Answer from the drawing. Dimensions are ordinates in mm from the lowest x, y and z of the part. A direction names the side the tool comes from. Round coordinates to 2 decimals unless told otherwise and drop trailing zeros. Write each loop counter-clockwise with the first axis right and the second up, starting at its lowest first coordinate (ties: lowest second). Pieces come first, ordered by that corner, then holes.
1. Find section A-A (x = 45). Write down the section's boundary in (y, z), and give its area (3 significant figures).
2. Find section D-D (z = 16). Write down the section's boundary in (x, y), and give its area (3 significant figures).
3. Determine the mould class of the marked faces 6, 7 and 8 for opening direction Z: pulls with the +Z half, pulls with the -Z half, needs draft (parallel to the pull), parting line crosses it, or undercut.
4. Find section B-B (y = 10). Write down the section's boundary in (x, z), and give its area (3 significant figures).
5. Flat-ended cylindrical pins translate along their axes: pin 1 Ø11 at (x, z) = (48, 37) entering from +Y; pin 2 Ø1 at (x, z) = (13.5, 14.5) entering from -Y; pin 3 Ø8 at (x, z) = (45.5, 33) entering from -Y; pin 4 Ø12 at (x, z) = (56.5, 17.5) entering from -Y. Find the tip coordinate at first contact, or state that the pin passes through.
6. Find section C-C (z = 34). Write down the section's boundary in (x, y).
7. Straight lines are drawn through the part: probe 1 along Z at (x, y) = (36, 8); probe 2 along X at (y, z) = (7.75, 8.5); probe 3 along X at (y, z) = (16.75, 16). For each, find the intervals that lie inside material, in ascending order.
8. A tool of negligible diameter and unlimited length cuts with its end or side. For the marked faces 1, 2, 3, 4 and 5, from which of +Z, -Z, +X, -X, +Y, -Y can it reach the whole face along a straight path? Write none if from no direction.
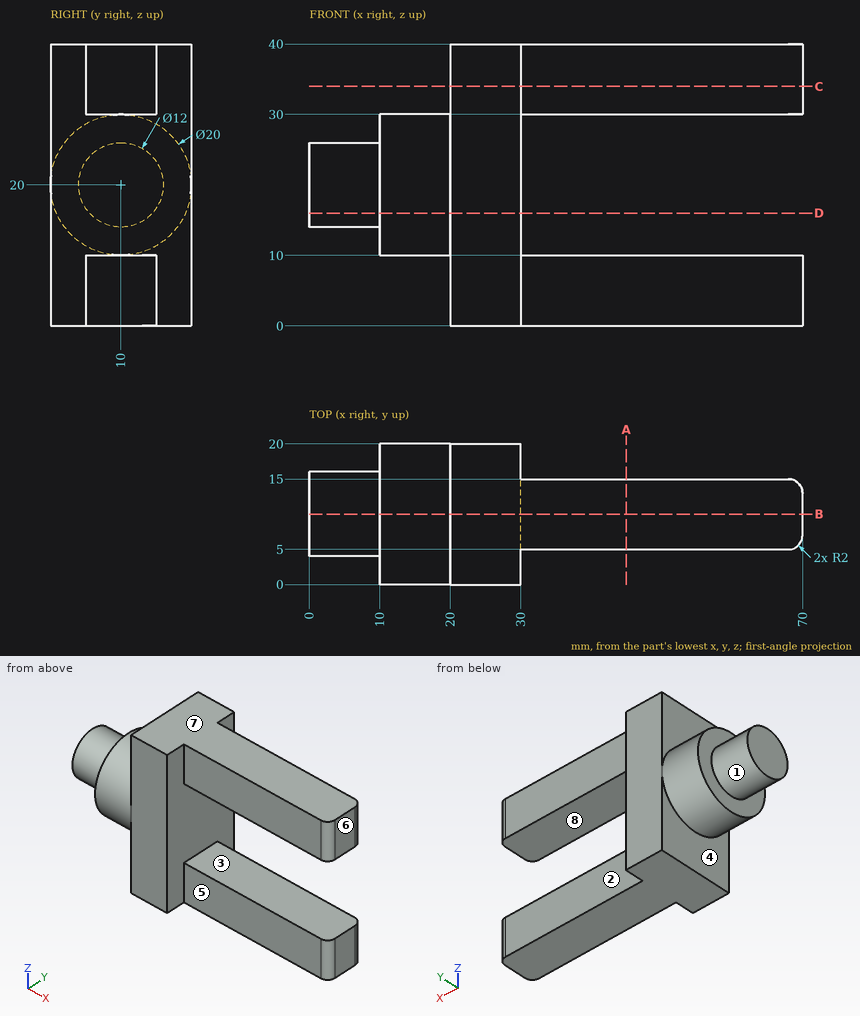
Worked answers:
1. outline: (5, 0) - (15, 0) - (15, 10) - (5, 10) - close; (5, 30) - (15, 30) - (15, 40) - (5, 40) - close
1. area: 200 mm2
2. outline: (0, 5.53) - (10, 5.53) - (10, 0.83) - (20, 0.83) - (20, 0) - (30, 0) - (30, 20) - (20, 20) - (20, 19.17) - (10, 19.17) - (10, 14.47) - (0, 14.47) - close
2. area: 473 mm2
3. face 6: needs draft
3. face 7: pulls with the +Z half
3. face 8: undercut
4. outline: (0, 14) - (10, 14) - (10, 10) - (20, 10) - (20, 0) - (70, 0) - (70, 10) - (30, 10) - (30, 30) - (70, 30) - (70, 40) - (20, 40) - (20, 30) - (10, 30) - (10, 26) - (0, 26) - close
4. area: 1,520 mm2
5. pin 1: stops at y = 15
5. pin 2: stops at y = 1.34
5. pin 3: stops at y = 5
5. pin 4: passes through
6. outline: (20, 0) - (30, 0) - (30, 5) - (68, 5) arc R2 ccw to (70, 7) - (70, 13) arc R2 ccw to (68, 15) - (30, 15) - (30, 20) - (20, 20) - close
7. probe 1: z = 0 to 10, 30 to 40
7. probe 2: x = 20 to 70
7. probe 3: x = 10 to 30
8. face 1: -X
8. face 2: +Z, -Z, +X, +Y
8. face 3: +X, +Y, -Y
8. face 4: -Z, -X
8. face 5: +Z, -Z, +X, -Y
